from build123d import *

# Parameters (mm, degrees)
PAD_DEPTH            = 10
SKETCH_R             = 1.6
PAD001_DEPTH         = 6
SKETCH004_R          = 2.5
POCKET_DEPTH         = 27.372693
SKETCH005_R          = 1.6
POCKET001_DEPTH      = 6.001
POCKET001_DEPTH_BACK = -6.001


with BuildPart() as part:
    # Sketch003 → Pad (new body)
    with BuildSketch(Plane.XZ):
        with BuildLine():
            Line((13.253575, -6), (-11.746425, -6))
            Line((-11.746425, -2.8), (-11.746425, -6))
            Line((-1.746425, -2.8), (-11.746425, -2.8))
            ThreePointArc((-1.746425, -2.8), (3.3, 0), (-1.746425, 2.8))
            Line((-1.746425, 2.8), (-11.746425, 2.8))
            Line((-11.746425, 2.8), (-11.746425, 6))
            Line((7.253575, 6), (-11.746425, 6))
            ThreePointArc((13.253575, 0), (11.496216, 4.242641), (7.253575, 6))
            Line((13.253575, 0), (13.253575, -6))
        make_face()
    extrude(amount=PAD_DEPTH)

    # Sketch → Pad001 (join)
    with BuildSketch(Plane.XY):
        Polygon((13.253575, -10), (20.324643, -17.071068), (30.324643, -17.071068), (34.517031, -12.87868), (17.445963, 4.192388), (13.253575, 0), align=None)
        with Locations((17.445963, -0.807612)):
            Circle(SKETCH_R, mode=Mode.SUBTRACT)
        with Locations((29.517031, -12.87868)):
            Circle(SKETCH_R, mode=Mode.SUBTRACT)
    extrude(amount=-PAD001_DEPTH)

    # Sketch004 (on DatumPlane) → Pocket (cut, through all)
    with BuildSketch(Plane(origin=(0, 0, 3.5), x_dir=(0, 0, -1), z_dir=(-0.707107, -0.707107, 0))):
        with Locations((3.5, 21.442761)):
            Circle(SKETCH004_R)
    extrude(amount=-POCKET_DEPTH, mode=Mode.SUBTRACT)

    # Sketch005 → Pocket001 (cut, two sides)
    with BuildSketch(Plane.XY) as pocket001_sk:
        with Locations((-7, -5)):
            Circle(SKETCH005_R)
    extrude(amount=-POCKET001_DEPTH, mode=Mode.SUBTRACT)
    extrude(pocket001_sk.sketch, amount=-POCKET001_DEPTH_BACK, mode=Mode.SUBTRACT)


solid = part.part
Read the model definition and answer for the solid it produces. Units are mm, in the model's axes. A direction names the side the tool comes from. Coordinates: 2 decimals unless noted, no trailing zeros. Loops run counter-clockwise (first coordinate to the right, second up) from the corner with the lowest first, then second, coordinate; pieces in that order, holes last. Notation, with made-up numbers: (85.25, -31) -> (121.25, -31) arc R13 cw to (121.25, -25) -> close; hole circle Ø11 at (-34.5, 73.25). An arc over 180 degrees is marked (long way). Write item = value, one per line. Start each with the question number.
1) The part is cut by section C-C, the plane x = -7.5. Determine the outline of the cut face in (y, z), plus the area to 3 significant figures.
2) For faces 5 (the face through (-5.6, -3.8, 2.8)), 6 (the face through (17, -4, 0)), 7 (the face through (4, -10, 0)), determine the directions among +Z, -Z, +X, -X, +Y, -Y from which every point of the face is accessible in a straight line to the end or side of a thin tool.
3) The part is cut by section D-D, the plane y = -4.5. State how many separate pieces and enclosed holes the cut face has, plus the area to 3 significant figures.
4) The part is cut by section A-A, the plane z = -0.5. Determine the outline of the cut face in (x, y), plus the area to 3 significant figures.
5) The part is cut by section B-B, the plane x = 0. Determine the outline of the cut face in (y, z), plus the area to 3 significant figures.
6) Find the intervals of material crossed by L1, parallel to Y at x = -7, z = -4.7; L2, parallel to Y at x = -4.5, z = -3.5; L3, parallel to X at y = -14.25, z = -0.25, in increasing order. Write a range as from..to.
7) The mould has two halves that part along Y. Classify faces 1 (the face through (4, 0, 0)), 2 (the face through (21.3, -9, -2.5)), 3 (the face through (-8.6, -4.93, -4.38)), 4 (the face through (-5.6, -3.8, -2.8)): pulls with the +Y half, pulls with the -Y half, needs draft (parallel to the pull), parting line crosses it, or undercut.
8) Given P1, Ø5, axis at x = 29.52, y = -12.88, coming from the +Z side; P2, Ø1.5, axis at x = 23, y = -7, coming from the +Z side; P3, Ø3, axis at x = 11.5, z = 0, coming from the -Y side, each flat-ended and moving along its own axis, determine where each tip first touches the part or whether it passes through.
Result:
q1.outline = (-10, -6) -> (-6.52, -6) -> (-6.52, -2.8) -> (-10, -2.8) -> close; (-10, 2.8) -> (-6.52, 2.8) -> (-6.52, 6) -> (-10, 6) -> close; (-3.48, -6) -> (0, -6) -> (0, -2.8) -> (-3.48, -2.8) -> close; (-3.48, 2.8) -> (0, 2.8) -> (0, 6) -> (-3.48, 6) -> close
q1.area = 44.5 mm²
q2.face_5 = -X, +Y, -Y
q2.face_6 = +Z, +X, +Y, -Y
q2.face_7 = +Z, -Z, -X, -Y
q3.separate_pieces = 3
q3.enclosed_holes = 0
q3.area = 258 mm²
q4.outline = (3.26, -10) -> (13.25, -10) -> (15.06, -11.8) -> (24.25, -2.61) -> (17.45, 4.19) -> (13.25, 0) -> (3.26, 0) -> close; (18.52, -15.27) -> (20.32, -17.07) -> (30.32, -17.07) -> (34.52, -12.88) -> (27.71, -6.08) -> close; hole circle Ø3.2 at (17.45, -0.81); hole circle Ø3.2 at (29.52, -12.88)
q4.area = 284 mm²
q5.outline = (-10, -6) -> (0, -6) -> (0, -3.3) -> (-10, -3.3) -> close; (-10, 3.3) -> (0, 3.3) -> (0, 6) -> (-10, 6) -> close
q5.area = 54.0 mm²
q6.L1 = -10..-6.6, -3.4..0
q6.L2 = -10..0
q6.L3 = 19.59..28.69, 30.34..33.15
q7.face_1 = pulls with the +Y half
q7.face_2 = undercut
q7.face_3 = undercut
q7.face_4 = needs draft
q8.P1 = 0
q8.P2 = -2.3
q8.P3 = -10
